Source: CAD feature listing. Evaluate the final solid. Frame: model axes, mm. A direction names the side the tool comes from. Round coordinates to 2 decimals unless told otherwise and drop trailing zeros. Write each loop counter-clockwise with the first axis right and the second up, starting at its lowest first coordinate (ties: lowest second). Pieces come first, ordered by that corner, then holes. Notation, with made-up numbers: M 55,-21.5 L 83,-21.5 A21 cw 83,-7.5 Z; hole C 21.25,56 d4. An arc over 180 degrees is marked long. Use a Markdown table: item, result.
```python
from build123d import *

# Parameters (mm, degrees)
SKETCH_1_W          = 40
SKETCH_1_H          = 24
SKETCH_1_R          = 2
EXTRUDE_1_DEPTH     = 3
SKETCH_2_W          = 20
SKETCH_2_H          = 6
EXTRUDE_2_DEPTH     = 25
SKETCH_3_R          = 7.9375
CUT_EXTRUDE_1_DEPTH = 10
EXTRUDE_4_DEPTH     = 6
SKETCH_5_R          = 8
CUT_EXTRUDE_2_DEPTH = 6


with BuildPart() as part:
    # 草图1 → 凸台-拉伸1 (new body)
    with BuildSketch(Plane(origin=(0, 0, 0), x_dir=(1, 0, 0), z_dir=(0, 1, 0))):
        Rectangle(SKETCH_1_W, SKETCH_1_H)
        with Locations((-14.8, -7.5)):
            Circle(SKETCH_1_R, mode=Mode.SUBTRACT)
        with Locations((14.8, -7.5)):
            Circle(SKETCH_1_R, mode=Mode.SUBTRACT)
        with Locations((-14.8, 7.5)):
            Circle(SKETCH_1_R, mode=Mode.SUBTRACT)
        with Locations((14.8, 7.5)):
            Circle(SKETCH_1_R, mode=Mode.SUBTRACT)
    extrude(amount=EXTRUDE_1_DEPTH)

    # 草图2 → 凸台-拉伸2 (add)
    with BuildSketch(Plane(origin=(0, 3, 0), x_dir=(1, 0, 0), z_dir=(0, 1, 0))):
        Rectangle(SKETCH_2_W, SKETCH_2_H)
    extrude(amount=EXTRUDE_2_DEPTH)

    # 草图3 → 切除-拉伸1 (cut)
    with BuildSketch(Plane.XY.offset(3)):
        with Locations((0, 17)):
            Circle(SKETCH_3_R)
    extrude(amount=-CUT_EXTRUDE_1_DEPTH, mode=Mode.SUBTRACT)

    # 草图4 → 凸台-拉伸4 (add)
    with BuildSketch(Plane.XY.offset(3)):
        Polygon((-15, 32), (-15, 3), (-10, 3), (-10, 28), (10, 28), (10, 3), (15, 3), (15, 32), align=None)
    extrude(amount=-EXTRUDE_4_DEPTH)

    # 草图5 → 切除-拉伸2 (cut)
    with BuildSketch(Plane.XY.offset(3)):
        with Locations((0, 17)):
            Circle(SKETCH_5_R)
    extrude(amount=-CUT_EXTRUDE_2_DEPTH, mode=Mode.SUBTRACT)


solid = part.part
```
Q1. Section B-B on y = 17. Return loops of the section in (x, z).
Results are:
| item | result |
|---|---|
| outline | M -15,-3 L -8,-3 L -8,3 L -15,3 Z; M 8,-3 L 15,-3 L 15,3 L 8,3 Z |
Q2. Section D-D on x = -14. Return loops of the section in (y, z), plus the area to 3 significant figures.
Results are:
| item | result |
|---|---|
| outline | M 0,-12 L 3,-12 L 3,-9.33 L 0,-9.33 Z; M 0,-5.67 L 3,-5.67 L 3,-3 L 32,-3 L 32,3 L 3,3 L 3,5.67 L 0,5.67 Z; M 0,9.33 L 3,9.33 L 3,12 L 0,12 Z |
| area | 224 mm^2 |
Q3. Mould query, pull axis Z, two halves, no side actions, for faces 5 (the cylindrical face through (12.802, 1.479, 7.412)), 6 (the cylindrical face through (-13.725, 1.479, -9.186)), 7 (the flat face through (0, 1, 12)), 8 (the flat face through (-20, 1, 0)). Classes: +Z half, -Z half, draft (parallel to the pull), parting line (faces both ways), or undercut.
Results are:
| item | result |
|---|---|
| face 5 | undercut |
| face 6 | undercut |
| face 7 | +Z half |
| face 8 | draft |
Q4. Section C-C on x = 0. Return loops of the section in (y, z).
Results are:
| item | result |
|---|---|
| outline | M 0,-12 L 3,-12 L 3,-3 L 9,-3 L 9,3 L 3,3 L 3,12 L 0,12 Z; M 25,-3 L 32,-3 L 32,3 L 25,3 Z |
Q5. Line query: L1, parallel to X at y = 1.65, z = 7.5; L2, parallel to Z at x = 14.8, y = 1.2; L3, parallel to Z at x = 14, y = 2. Output: solid intervals per line, ascending.
Results are:
| item | result |
|---|---|
| L1 | -20 to -16.8, -12.8 to 12.8, 16.8 to 20 |
| L2 | -12 to -9.5, -5.5 to 5.5, 9.5 to 12 |
| L3 | -12 to -9.33, -5.67 to 5.67, 9.33 to 12 |
Q6. Reachability of faces 1 (the flat face through (-15, 18, 0)), 2 (the flat face through (-7, 11, -3)), 3 (the flat face through (15, 17, 0)), 4 (the flat face through (-7, 11, 3)) from +Z, -Z, +X, -X, +Y, -Y: full face, straight path, thin tool, end or side. Return the list, or none.
Results are:
| item | result |
|---|---|
| face 1 | +Z, -Z, -X, +Y |
| face 2 | -Z, +X, -X, +Y |
| face 3 | +Z, -Z, +X, +Y |
| face 4 | +Z, +X, -X, +Y |
Q7. First-contact query: pin 1 Ø6 at (y, z) = (13, 5) entering from +X; pin 2 Ø2 at (y, z) = (3.5, 4) entering from -X; pin 3 Ø6 at (x, y) = (-7.5, 23.5) entering from -Z; pin 4 Ø12 at (y, z) = (19, -3.5) entering from -X. Flat tips, straight axial feed; report the tip coordinate or a pass-through.
Results are:
| item | result |
|---|---|
| pin 1 | x = 15 |
| pin 2 | x = -20 |
| pin 3 | z = -3 |
| pin 4 | x = -15 |
Q8. Section A-A on z = -7.5. Return loops of the section in (x, y), plus the area to 3 significant figures.
Results are:
| item | result |
|---|---|
| outline | M -20,0 L -16.8,0 L -16.8,3 L -20,3 Z; M -12.8,0 L 12.8,0 L 12.8,3 L -12.8,3 Z; M 16.8,0 L 20,0 L 20,3 L 16.8,3 Z |
| area | 96.0 mm^2 |
